from build123d import *

# Parameters (mm, degrees)
F0_R     = 15
F1_DEPTH = 75
F2_R     = 5
F3_DEPTH = 15
F5_DEPTH = 10
F7_DEPTH = 10


with BuildPart() as f1:
    # F0 (on Top) → F1 (new body)
    with BuildSketch(Plane.XY):
        with BuildLine():
            Line((-50, -25), (0, -25))
            ThreePointArc((0, -25), (17.6776695297, -17.6776695297), (25, 0))
            Line((25, 0), (25, 10.3068929166))
            Line((25, 10.3068929166), (70, 10.3068929166))
            Line((70, 10.3068929166), (70, 25))
            Line((70, 25), (0, 25))
            ThreePointArc((0, 25), (-17.6776695297, 17.6776695297), (-25, 0))
            Line((-25, 0), (-25, -15))
            Line((-25, -15), (-40, -15))
            Line((-40, -15), (-40, 50))
            Line((-40, 50), (-50, 50))
            Line((-50, 50), (-50, -25))
        make_face()
        Circle(F0_R, mode=Mode.SUBTRACT)
    extrude(amount=F1_DEPTH)

    # F2 (on face) → F3 (cut)
    with BuildSketch(Plane(origin=(0, 25, 0), x_dir=(-1, 0, 0), z_dir=(0, 1, 0))):
        with Locations((-55, 20)):
            Circle(F2_R)
        with Locations((-55, 55)):
            Circle(F2_R)
    extrude(amount=-F3_DEPTH, mode=Mode.SUBTRACT)

    # F4 (on face) → F5 (cut)
    with BuildSketch(Plane.YZ.offset(-40)):
        with BuildLine():
            ThreePointArc((25, 40), (22.0710678119, 47.0710678119), (15, 50))
            ThreePointArc((15, 50), (7.9289321881, 32.9289321881), (25, 40))
        make_face()
    extrude(amount=-F5_DEPTH, mode=Mode.SUBTRACT)

    # F6 (on face) → F7 (cut)
    with BuildSketch(Plane.YZ.offset(-40)):
        Polygon((35, 75), (50, 60), (50, 75), align=None)
        Polygon((50, 0), (50, 15), (35, 0), align=None)
    extrude(amount=-F7_DEPTH, mode=Mode.SUBTRACT)


solid = f1.part
Can you work these out from the model? Positions are in its coordinate system, mm. A direction names the side the tool comes from. Round coordinates to 2 decimals unless told otherwise and drop trailing zeros. Write each loop counter-clockwise with the first axis right and the second up, starting at its lowest first coordinate (ties: lowest second). Pieces come first, ordered by that corner, then holes. Notation, with made-up numbers: M 6,-34 L 55,-34 A27 cw 55,-8 Z; hole C -34.5,64.25 d9. An arc over 180 degrees is marked long. Use CSV: the item, a comma, the result in double quotes.
(1) Imagine slicing it at C-C (z = 63.5). Write out the boundary of the cut face in (x, y), plus the area to 3 significant figures.
Check values:
outline,"M -50,-25 L 0,-25 A25 ccw 25,0 L 25,10.31 L 70,10.31 L 70,25 L 0,25 A25 ccw -25,0 L -25,-15 L -40,-15 L -40,46.5 L -50,46.5 Z; hole C 0,0 d30"
area,"3,050 mm^2"
(2) We'd pull the mould along Z, two halves only. Please class faces 1 (the flat face through (-45, 43, 8)), 2 (the cylindrical face through (59, 18, 17)), 3 (the cylindrical face through (-14.985, 0.66, 36.975)): +Z half, -Z half, draft (parallel to the pull), parting line (faces both ways), or undercut.
Check values:
face 1,"-Z half"
face 2,"undercut"
face 3,"draft"
(3) I need wall thicknesses on line 1 along Z through (x, y) = (55, 20.5); line 2 along X through (y, z) = (-12, 70); line 3 along Z through (x, y) = (-45.25, 15). Which ranges of each line are inside material? Lowest first, please.
Check values:
line 1,"0 to 15, 25 to 50, 60 to 75"
line 2,"-50 to -40, -25 to -9, 9 to 21.93"
line 3,"0 to 30, 50 to 75"
(4) Imagine slicing it at A-A (z = 55). Write out the boundary of the cut face in (x, y), plus the area to 3 significant figures.
Check values:
outline,"M -50,-25 L 0,-25 A25 ccw 25,0 L 25,10.31 L 50,10.31 L 50,25 L 0,25 A25 ccw -25,0 L -25,-15 L -40,-15 L -40,50 L -50,50 Z; M 60,10.31 L 70,10.31 L 70,25 L 60,25 Z; hole C 0,0 d30"
area,"2,940 mm^2"
(5) On a 3-axis mill with a long thin cutter (end or side, diameter ignored), from which of +Z, -Z, +X, -X, +Y, -Y can I reach the whole of each face in a straight line? I mean faces 4 (the flat face through (-40, 17, 29)), 5 (the flat face through (47, 10.307, 37)), 6 (the flat face through (35, 25, 37)), 7 (the flat face through (-45, 50, 37)). Say none if no direction works.
Check values:
face 4,"+Z, -Z, +Y"
face 5,"+Z, -Z, +X, -Y"
face 6,"+Z, -Z, +X, +Y"
face 7,"+Z, -Z, +X, -X, +Y"
(6) Imagine slicing it at B-B (x = 55). Write out the boundary of the cut face in (y, z), plus the area to 3 significant figures.
Check values:
outline,"M 10.31,0 L 25,0 L 25,15 L 10.31,15 Z; M 10.31,25 L 25,25 L 25,50 L 10.31,50 Z; M 10.31,60 L 25,60 L 25,75 L 10.31,75 Z"
area,"808 mm^2"
(7) I'm going to push flat-ended pins straight in: pin 1 (11.5 mm diameter, centred on x = 55, z = 20, fed in from -Y); pin 2 (2 mm diameter, centred on x = 25.5, z = 18.5, fed in from +Y); pin 3 (1.5 mm diameter, centred on y = -6.5, z = 36, fed in from +X). Where does each tip first touch, or does it pass through?
Check values:
pin 1,"y = 10.31"
pin 2,"y = 25"
pin 3,"x = 24.33"
(8) Imagine slicing it at D-D (x = 11). Write out the boundary of the cut face in (y, z), plus the area to 3 significant figures.
Check values:
outline,"M -22.45,0 L -10.2,0 L -10.2,75 L -22.45,75 Z; M 10.2,0 L 25,0 L 25,75 L 10.2,75 Z"
area,"2,030 mm^2"
